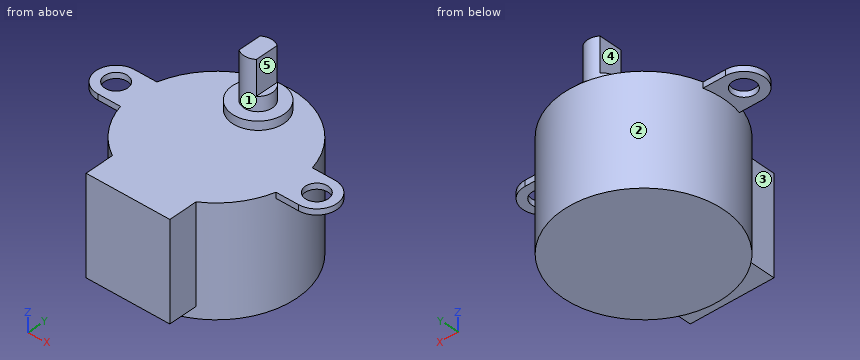
Autodesk Inventor part; units mm, degrees
ref_plane "YZ Plane" through (0, 0, 0) normal (1, 0, 0) x (0, 1, 0)
ref_plane "XZ Plane" through (0, 0, 0) normal (0, 1, 0) x (-1, 0, 0)
ref_plane "XY Plane" through (0, 0, 0) normal (0, 0, 1) x (1, 0, 0)
sketch "Náčrt1" plane through (0, 0, 0) normal (0, 0, 1) x (1, 0, 0)
  circle A0 centre (0, 0) radius 14
  dimension "d0" = 28
extrude "Vysunutí1" add sketch "Náčrt1" along normal blind 19
sketch "Náčrt2" plane through (0, 0, 19) normal (0, 0, 1) x (1, 0, 0)
  circle A0 centre (17.5, 0) radius 2
  circle A1 centre (-17.5, 0) radius 2
  line L0 (-17.5, 0) -> (17.5, 0) construction
  line L1 (-17.5, -3.5) -> (17.5, -3.5)
  line L2 (17.5, 3.5) -> (-17.5, 3.5)
  arc A2 (-17.5, 3.5) -> (-17.5, -3.5) centre (-17.5, 0) ccw
  arc A3 (17.5, -3.5) -> (17.5, 3.5) centre (17.5, 0) ccw
  point P0 (0, 0)
  point P1 (0, 0)
  dimension "d3" = 4
  dimension "d4" = 4
  dimension "d5" = 35
  dimension "d9" = 17.5
  dimension "d10" = 7
extrude "Vysunutí2" add sketch "Náčrt2" against normal blind 1
sketch "Náčrt3" plane through (0, 0, 19) normal (0, 0, 1) x (1, 0, 0)
  circle A0 centre (0, 8) radius 4.5
  point P0 (0, 0)
  dimension "d13" = 9
  dimension "d14" = 8
extrude "Vysunutí3" add sketch "Náčrt3" along normal blind 1.5
sketch "Náčrt4" plane through (0, 8, 20.5) normal (0, 0, 1) x (1, 0, 0)
  circle A0 centre (0, 0) radius 2.5
  point P0 (0, -8)
  dimension "d17" = 5
extrude "Vysunutí4" add sketch "Náčrt4" along normal blind 8.5
sketch "Náčrt5" plane through (0, 8, 29) normal (0, 0, 1) x (1, 0, 0)
  line L0 (-1.5, -2.5) -> (1.5, -2.5)
  line L1 (1.5, -2.5) -> (1.5, 2.5)
  line L2 (1.5, 2.5) -> (-1.5, 2.5)
  line L3 (-1.5, 2.5) -> (-1.5, -2.5)
  line L4 (-1.5, -2.5) -> (1.5, 2.5) construction
  line L5 (1.5, -2.5) -> (-1.5, 2.5) construction
  line L6 (-3, -3) -> (3, -3)
  line L7 (3, -3) -> (3, 3)
  line L8 (3, 3) -> (-3, 3)
  line L9 (-3, 3) -> (-3, -3)
  line L10 (-3, -3) -> (3, 3) construction
  line L11 (3, -3) -> (-3, 3) construction
  point P0 (0, -8)
  point P1 (0, 0)
  point P2 (0, 0)
  dimension "d20" = 3
  dimension "d21" = 5
  dimension "d22" = 6
  dimension "d23" = 6
extrude "Vysunutí5" cut sketch "Náčrt5" against normal blind 6
sketch "Náčrt6" plane through (0, 0, 19) normal (0, 0, 1) x (1, 0, 0)
  line L0 (-7.3, 17) -> (7.3, 17)
  line L1 (7.3, 17) -> (7.3, -17)
  line L2 (7.3, -17) -> (-7.3, -17)
  line L3 (-7.3, -17) -> (-7.3, 17)
  line L4 (-7.3, 17) -> (7.3, -17) construction
  line L5 (7.3, 17) -> (-7.3, -17) construction
  line L6 (-7.3, -8.0625) -> (7.3, -8.0625)
  point P0 (0, 0)
  dimension "d26" = 14.6
  dimension "d27" = 34
extrude "Vysunutí6" add sketch "Náčrt6" against normal blind 17 contours L6 L1 L2 L3
properties part number "StepperMotor"
Check sheet for the modelled part. Datum: model origin and axes. Units: mm. Face numbers are marked on the shaded views. A direction names the side the tool comes from. Coordinates: 2 decimals unless noted, no trailing zeros. Loops run counter-clockwise (first coordinate to the right, second up) from the corner with the lowest first, then second, coordinate; pieces in that order, holes last. Notation, with made-up numbers: (73, 21.5) -> (89, 21.5) arc R23 ccw to (89, 55.5) -> close; hole circle Ø3 at (57, 40). An arc over 180 degrees is marked (long way). Write item = value, one per line. Start each with the question number.
1. Section check C-C on x = 16. Record the cut outline in (y, z), then the cut area to 3 significant figures.
2. Section check B-B on x = 0. Record the cut outline in (y, z), then the cut area to 3 significant figures.
3. Depth check by flat-ended pin: P1, Ø12, axis at y = -2, z = 11, coming from the -X side; P2, Ø6, axis at x = -16, y = -1, coming from the +Z side; P3, Ø5.5, axis at x = -19, y = 0.5, coming from the -Z side; P4, Ø1.1, axis at x = -2, y = 8.5, coming from the +Z side. Enter the tip coordinate at first touch or a pass-through.
4. Tool access check on the marked faces 1, 2, 3, 4 and 5. Record the directions out of +Z, -Z, +X, -X, +Y, -Y that give a thin tool (end or side, any length) a straight path to the whole face; none if there is none.
5. Material ranges on line 1 (Y direction, x = 17.5, z = 18.5); line 2 (Z direction, x = 5, y = -2.5); line 3 (X direction, y = -12, z = 14.75), recorded low to high.
6. Section check A-A on y = 0. Record the cut outline in (x, z).
7. Section check D-D on z = 20. Record the cut outline in (x, y).
Responses:
q1.outline = (-3.5, 18) -> (-1.32, 18) -> (-1.32, 19) -> (-3.5, 19) -> close; (1.32, 18) -> (3.5, 18) -> (3.5, 19) -> (1.32, 19) -> close
q1.area = 4.35 mm2
q2.outline = (-17, 2) -> (-14, 2) -> (-14, 0) -> (14, 0) -> (14, 19) -> (12.5, 19) -> (12.5, 20.5) -> (10.5, 20.5) -> (10.5, 29) -> (5.5, 29) -> (5.5, 20.5) -> (3.5, 20.5) -> (3.5, 19) -> (-17, 19) -> close
q2.area = 639 mm2
q3.P1 = -14
q3.P2 = 19
q3.P3 = 18
q3.P4 = 29
q4.face_1 = +Z
q4.face_2 = -Z
q4.face_3 = +Z, -Z, -X, -Y
q4.face_4 = +Z, -X, +Y, -Y
q4.face_5 = +Z, +X, +Y, -Y
q5.line_1 = -3.5 to -2, 2 to 3.5
q5.line_2 = 0 to 19
q5.line_3 = -7.3 to 7.3
q6.outline = (-21, 18) -> (-19.5, 18) -> (-19.5, 19) -> (-21, 19) -> close; (-15.5, 18) -> (-14, 18) -> (-14, 0) -> (14, 0) -> (14, 18) -> (15.5, 18) -> (15.5, 19) -> (-15.5, 19) -> close; (19.5, 18) -> (21, 18) -> (21, 19) -> (19.5, 19) -> close
q7.outline = circle Ø9 at (0, 8)
